For this review, take the finished solid that the model builds, in its own axes (mm). Round coordinates to 2 decimals unless told otherwise and drop trailing zeros. Order: outer loops, then holes, each group sorted by start corner. A loop starts at its lowest first (then second) coordinate and runs counter-clockwise, first axis right, second up. Notation, with made-up numbers: M 16.25,64.5 L 29.25,64.5 A16 cw 29.25,71.5 Z; hole C -24,3 d3. An arc over 180 degrees is marked long. Use a Markdown table: item, result.
from build123d import *

# Parameters (mm, degrees)
BOSS_EXTRUDE1_DEPTH     = 60
CUT_EXTRUDE1_DEPTH      = 61.889736409
CUT_EXTRUDE1_DEPTH_BACK = 61.889736409
SKETCH4_W               = 0.254
SKETCH4_H               = 0.381
LPATTERN2_COUNT         = 5
LPATTERN2_PITCH         = 25


with BuildPart() as part:
    # Sketch1 → Boss-Extrude1 (new, symmetric)
    with BuildSketch(Plane.XY):
        with BuildLine():
            Line((-4.85, 8), (-3.7, 8))
            Line((-3.7, 8), (-3.078681812, 7.4))
            Line((-3.078681812, 7.4), (3.078681812, 7.4))
            Line((3.078681812, 7.4), (3.7, 8))
            Line((3.7, 8), (4.85, 8))
            ThreePointArc((4.85, 8), (6.6, 6.25), (4.85, 4.5))
            Line((4.85, 4.5), (3.55, 4.5))
            Line((3.55, 4.5), (3.55, 2.41450816))
            Line((3.55, 2.41450816), (5.746, 1.146646968))
            ThreePointArc((5.746, 1.146646968), (5.931940905, 0.960706063), (6, 0.706706063))
            Line((6, 0.706706063), (6, 0.254))
            ThreePointArc((6, 0.254), (5.925605122, 0.074394878), (5.746, 0))
            Line((5.746, 0), (-5.746, 0))
            ThreePointArc((-5.746, 0), (-5.925605122, 0.074394878), (-6, 0.254))
            Line((-6, 0.254), (-6, 0.706706063))
            ThreePointArc((-6, 0.706706063), (-5.931940905, 0.960706063), (-5.746, 1.146646968))
            Line((-5.746, 1.146646968), (-3.55, 2.41450816))
            Line((-3.55, 2.41450816), (-3.55, 4.5))
            Line((-3.55, 4.5), (-4.85, 4.5))
            ThreePointArc((-4.85, 4.5), (-6.6, 6.25), (-4.85, 8))
        make_face()
    extrude(amount=BOSS_EXTRUDE1_DEPTH, both=True)

    # Sketch4 → Cut-Extrude1 (cut, two sides: drawn at the far end of the back side and taken through both)
    with BuildSketch(Plane.XY.offset(-CUT_EXTRUDE1_DEPTH_BACK)):
        with Locations((5.873, 0.5969)):
            Rectangle(SKETCH4_W, SKETCH4_H)
    extrude(amount=CUT_EXTRUDE1_DEPTH + CUT_EXTRUDE1_DEPTH_BACK, mode=Mode.SUBTRACT)

    # Sketch2 → Cut-Revolve1 (revolve, cut)
    with BuildSketch(Plane(origin=(0, 0, 0), x_dir=(0, 0, -1), z_dir=(1, 0, 0)), mode=Mode.PRIVATE) as cut_revolve1_sk:
        Polygon((-53, 7.4), (-53, 4.5), (-51.75, 4.5), (-51.75, 0), (-50, 0), (-50, 7.4), (-50, 8), (-53, 8), align=None)
    cut_revolve1 = revolve(cut_revolve1_sk.sketch.rotate(Axis((0, 0, 50), (0, 1, 0)), 180), axis=Axis((0, 0, 50), (0, 1, 0)), mode=Mode.SUBTRACT)

    # LPattern2: Cut-Revolve1 ×5
    with Locations(*[(0, 0, -i * LPATTERN2_PITCH) for i in range(1, LPATTERN2_COUNT)]):
        add(cut_revolve1, mode=Mode.SUBTRACT)


solid = part.part
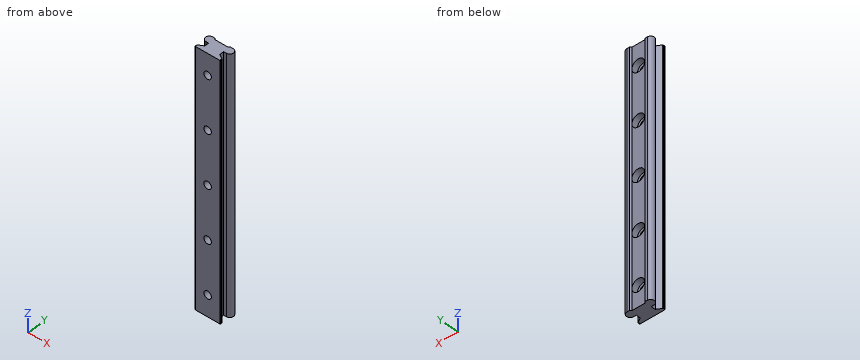
Q1. Clearance check with flat-ended pins moving along their axes: pin 1 (0.5 mm diameter, centred on y = 0.5, z = -5.5, fed in from -X); pin 2 (1.8 mm diameter, centred on x = 1, z = 26, fed in from +Y); pin 3 (3 mm diameter, centred on x = 1, z = -12.5, fed in from +Y). State where each tip first meets the part, or that it passes through.
Determined:
| item | result |
|---|---|
| pin 1 | stops at x = -6 |
| pin 2 | stops at y = 4.5 |
| pin 3 | stops at y = 7.4 |
Q2. Add section B-B (z = 37). Write out the cut boundary in (x, y), then the cut area to 3 significant figures.
Determined:
| item | result |
|---|---|
| outline | M -6,0.25 A0.25 ccw -5.75,0 L 5.75,0 A0.25 ccw 6,0.25 L 6,0.41 L 5.75,0.41 L 5.75,0.79 L 5.99,0.79 A0.51 ccw 5.75,1.15 L 3.55,2.41 L 3.55,4.5 L 4.85,4.5 A1.75 ccw 4.85,8 L 3.7,8 L 3.08,7.4 L -3.08,7.4 L -3.7,8 L -4.85,8 A1.75 ccw -4.85,4.5 L -3.55,4.5 L -3.55,2.41 L -5.75,1.15 A0.51 ccw -6,0.71 Z |
| area | 79.7 mm^2 |
Q3. Wall thickness on line 1 along X through (y, z) = (6.25, -50); line 2 along X through (y, z) = (3.2, 50); line 3 along Z through (x, y) = (1.75, 6.75): over which ranges is each line inside the solid? List them lowest first. Write a range as [from, to].
Determined:
| item | result |
|---|---|
| line 1 | x = [-6.6, -3], [3, 6.6] |
| line 2 | x = [-3.55, -1.75], [1.75, 3.55] |
| line 3 | z = [-60, -52.44], [-47.56, -27.44], [-22.56, -2.44], [2.44, 22.56], [27.44, 47.56], [52.44, 60] |
